Read the model definition and answer for the solid it produces. Units are mm, in the model's axes. A direction names the side the tool comes from. Round coordinates to 2 decimals unless told otherwise and drop trailing zeros. Write each loop counter-clockwise with the first axis right and the second up, starting at its lowest first coordinate (ties: lowest second). Pieces come first, ordered by that corner, then holes. Notation, with made-up numbers: (52.5, 21) - (101.5, 21) arc R17 ccw to (101.5, 35) - close; hole circle Ø5 at (89.5, -14.75). An arc over 180 degrees is marked (long way). Answer as CSV lines item,"result". Start each with the question number.
1) Which of the six approach directions +Z, -Z, +X, -X, +Y, -Y give full straight-line access (tool end or side, diameter ignored) to faces 5 (the flat face through (302.92, -6.26, 60.5)), 6 (the flat face through (353.18, -6.261, 44.006)), 7 (the flat face through (322, -6, 49.985))?
2) Find section C-C on z = 61.99. State how many separate pieces and enclosed holes the cut face has, then the cut area to 3 significant figures.
3) Find section B-B on z = 29.74. Determine the outline of the cut face in (x, y) (3 decimals).
4) Find section D-D on x = 215.5. Determine the outline of the cut face in (y, z).
5) Consider line 1 along Z through (x, y) = (322, -5) (3 decimals); line 2 along X through (y, z) = (-10, 21.5); line 3 along Z through (x, y) = (325, -2) (1 decimal). Determine where each line is inside the solid, lowest interval first.
6) Find section A-A on x = 137. Determine the outline of the cut face in (y, z).
7) Each of these flat-tipped pins is pushed along its axis until it touches: pin 1 (1.5 mm diameter, centred on y = -4.5, z = 54.5, fed in from +X); pin 2 (1 mm diameter, centred on y = -10.5, z = 32.5, fed in from -X); pin 3 (6 mm diameter, centred on y = -10, z = 48.5, fed in from +X); pin 4 (9 mm diameter, centred on x = 230, z = 61.99, fed in from +Y). Where does it stop, or does it pass through?
8) For a pull along Z with two mould halves and no side action, classify faces 1 (the flat face through (181, -12.7, 29)), 2 (the flat face through (14.45, -6.26, 44.74)), 3 (the cylindrical face through (14.755, -6.261, 29.295)), 4 (the cylindrical face through (234.78, -6.26, 63.49)) as +Z half, -Z half, draft (parallel to the pull), parting line (faces both ways), or undercut.
from build123d import *

# Parameters (mm, degrees)
F0_R     = 6.01
F0_R_2   = 5.01
F1_DEPTH = 12.7


with BuildPart() as f1:
    # F0 (on Front) → F1 (new body)
    with BuildSketch(Plane.XZ):
        with BuildLine():
            Line((183.5, 0), (367, 0))
            ThreePointArc((367, 0), (377.016632, 6.473352), (375.248216, 18.267838))
            Line((375.248216, 18.267838), (330.485281, 70.475281))
            ThreePointArc((330.485281, 70.475281), (322.178418, 73.988674), (313.770763, 70.723823))
            Line((313.770763, 70.723823), (291.760312, 49.984999))
            ThreePointArc((291.760312, 49.984999), (276.005306, 43.731851), (260.2503, 49.984999))
            Line((260.2503, 49.984999), (238.227135, 70.725803))
            ThreePointArc((238.227135, 70.725803), (230, 73.99), (221.772865, 70.725803))
            Line((221.772865, 70.725803), (199.755006, 49.99))
            ThreePointArc((199.755006, 49.99), (183.5, 43.540666), (167.244994, 49.99))
            Line((167.244994, 49.99), (145.227135, 70.725803))
            ThreePointArc((145.227135, 70.725803), (137, 73.99), (128.772865, 70.725803))
            Line((128.772865, 70.725803), (106.7497, 49.984999))
            ThreePointArc((106.7497, 49.984999), (90.994694, 43.731851), (75.239688, 49.984999))
            Line((75.239688, 49.984999), (53.229237, 70.723823))
            ThreePointArc((53.229237, 70.723823), (44.821582, 73.988674), (36.514719, 70.475281))
            Line((36.514719, 70.475281), (-8.248216, 18.267838))
            ThreePointArc((-8.248216, 18.267838), (-10.016632, 6.473352), (0, 0))
            Line((0, 0), (183.5, 0))
        make_face()
        with Locations((0.00881, 10.999996)):
            Circle(F0_R, mode=Mode.SUBTRACT)
        with Locations((92, 11)):
            Circle(F0_R_2, mode=Mode.SUBTRACT)
        with BuildLine():
            ThreePointArc((183.5, 16), (188.5, 11), (183.5, 6))
            ThreePointArc((183.5, 6), (178.5, 11), (183.5, 16))
        make_face(mode=Mode.SUBTRACT)
        with BuildLine():
            Line((34.994694, 49.984999), (54.994694, 49.984999))
            ThreePointArc((54.994694, 49.984999), (75.239694, 29.739999), (54.994694, 9.494999))
            Line((54.994694, 9.494999), (34.994694, 9.494999))
            ThreePointArc((34.994694, 9.494999), (14.749694, 29.739999), (34.994694, 49.984999))
        make_face(mode=Mode.SUBTRACT)
        with BuildLine():
            ThreePointArc((147, 49.99), (167.245, 29.745), (147, 9.5))
            Line((147, 9.5), (127, 9.5))
            ThreePointArc((127, 9.5), (106.755, 29.745), (127, 49.99))
            Line((127, 49.99), (147, 49.99))
        make_face(mode=Mode.SUBTRACT)
        with Locations((275, 11)):
            Circle(F0_R_2, mode=Mode.SUBTRACT)
        with Locations((366.99119, 10.999996)):
            Circle(F0_R, mode=Mode.SUBTRACT)
        with BuildLine():
            Line((240, 9.5), (220, 9.5))
            ThreePointArc((220, 9.5), (199.755, 29.745), (220, 49.99))
            Line((220, 49.99), (240, 49.99))
            ThreePointArc((240, 49.99), (260.245, 29.745), (240, 9.5))
        make_face(mode=Mode.SUBTRACT)
        with BuildLine():
            ThreePointArc((332.005306, 49.984999), (352.250306, 29.739999), (332.005306, 9.494999))
            Line((332.005306, 9.494999), (312.005306, 9.494999))
            ThreePointArc((312.005306, 9.494999), (291.760306, 29.739999), (312.005306, 49.984999))
            Line((312.005306, 49.984999), (332.005306, 49.984999))
        make_face(mode=Mode.SUBTRACT)
        with Locations((45, 61.99)):
            Circle(F0_R_2, mode=Mode.SUBTRACT)
        with Locations((137, 61.99)):
            Circle(F0_R_2, mode=Mode.SUBTRACT)
        with Locations((230, 61.99)):
            Circle(F0_R_2, mode=Mode.SUBTRACT)
        with Locations((322, 61.99)):
            Circle(F0_R_2, mode=Mode.SUBTRACT)
    extrude(amount=F1_DEPTH)


solid = f1.part
Check values:
1,face 5,"+Z, +Y, -Y"
1,face 6,"+Z, +X, +Y, -Y"
1,face 7,"+Y, -Y"
2,separate pieces,"8"
2,enclosed holes,"0"
2,area,"1,220 mm^2"
3,outline,"(1.588, -12.7) - (14.75, -12.7) - (14.75, 0) - (1.588, 0) - close; (75.24, -12.7) - (106.755, -12.7) - (106.755, 0) - (75.24, 0) - close; (167.245, -12.7) - (199.755, -12.7) - (199.755, 0) - (167.245, 0) - close; (260.245, -12.7) - (291.76, -12.7) - (291.76, 0) - (260.245, 0) - close; (352.25, -12.7) - (365.412, -12.7) - (365.412, 0) - (352.25, 0) - close"
4,outline,"(-12.7, 0) - (0, 0) - (0, 10.01) - (-12.7, 10.01) - close; (-12.7, 49.48) - (0, 49.48) - (0, 64.82) - (-12.7, 64.82) - close"
5,line 1,"z = 0 to 9.495, 49.985 to 56.98, 67 to 73.99"
5,line 2,"x = -5.48 to 16.5, 73.49 to 108.51, 165.49 to 201.51, 258.49 to 293.51, 350.5 to 372.48"
5,line 3,"z = 0 to 9.5, 50 to 58, 66 to 73.6"
6,outline,"(-12.7, 0) - (0, 0) - (0, 9.5) - (-12.7, 9.5) - close; (-12.7, 49.99) - (0, 49.99) - (0, 56.98) - (-12.7, 56.98) - close; (-12.7, 67) - (0, 67) - (0, 73.99) - (-12.7, 73.99) - close"
7,pin 1,"stops at x = 344.83"
7,pin 2,"stops at x = 3.53"
7,pin 3,"stops at x = 351.9"
7,pin 4,"passes through"
8,face 1,"draft"
8,face 2,"+Z half"
8,face 3,"undercut"
8,face 4,"undercut"
